Autodesk Inventor part; units mm, degrees
ref_plane "YZ Plane" through (0, 0, 0) normal (1, 0, 0) x (0, 1, 0)
ref_plane "XZ Plane" through (0, 0, 0) normal (0, 1, 0) x (-1, 0, 0)
ref_plane "XY Plane" through (0, 0, 0) normal (0, 0, 1) x (1, 0, 0)
sketch "Sketch1" plane through (0, 0, 0) normal (0, 0, 1) x (1, 0, 0)
  line L0 (-99.06, 38.1) -> (-99.06, -38.1)
  circle A0 centre (-60.96, 0) radius 12.7
  circle A1 centre (99.06, 0) radius 1.27
  line L1 (-99.06, 38.1) -> (99.06, 38.1)
  line L2 (-99.06, -38.1) -> (99.06, -38.1)
  arc A2 (99.06, -38.1) -> (99.06, 38.1) centre (99.06, 0) ccw
  line L3 (-48.6633, 3.175) -> (-45.3613, 3.175)
  line L4 (-45.3613, 3.175) -> (-45.3613, -3.175)
  line L5 (-45.3613, -3.175) -> (-48.6633, -3.175)
  point P0 (0, 0)
  point P1 (-99.06, 0)
  point P2 (106.7321, -3.216)
  point P3 (113.0654, -3.216)
  point P4 (-45.3613, 0)
  point P5 (0, -38.1)
  dimension "d0" = 76.2
  dimension "d4" = 25.4
  dimension "d13" = 2.54
  dimension "d14" = 6.35
  dimension "d15" = 160.02
  dimension "d16" = 3.302
  dimension "d17" = 38.1
extrude "Extrusion2" add sketch "Sketch1" along normal blind 25.4
sketch "Sketch2" plane through (0, 0, 25.4) normal (0, 0, 1) x (1, 0, 0)
  arc A0 (-48.6633, 3.175) -> (-48.6633, -3.175) centre (-60.96, 0) ccw
  point P0 (0, 0)
  point P1 (-80.01, 19.05)
  point P2 (-41.91, 19.05)
  point P3 (-41.91, -19.05)
  point P4 (-80.01, -19.05)
  dimension "d20" = 38.1
  dimension "d21" = 38.1
  dimension "d22" = 19.05
  dimension "d23" = 19.05
hole "Hole1" at (-80.01, 19.05, 25.4) at (-41.91, 19.05, 25.4) at (-41.91, -19.05, 25.4) at (-80.01, -19.05, 25.4) direction (0, 0, -1) diameter 4.9784 depth 25.4 tip angle 118
sketch "Sketch4" plane through (0, 0, 25.4) normal (0, 0, 1) x (1, 0, 0)
  circle A0 centre (99.06, 0) radius 1.27
  point P0 (0, 0)
hole "Hole3" at (99.06, 0, 25.4) direction (0, 0, -1) diameter 10.5918 end through all
properties part number "Motor_Arm"
Geometry check sheet. Reference: the model listing, model coordinates, mm. Coordinates: 2 decimals unless noted, no trailing zeros. Order: outer loops, then holes, each group sorted by start corner. A loop starts at its lowest first (then second) coordinate and runs counter-clockwise, first axis right, second up.
Item 1: Section check B-B (x = -60.96). Enter the section's corners in (y, z).
Item 2: Scan lines: line 1 along X through (y, z) = (0, 15.75); line 2 along Y through (x, z) = (99.06, 7.75); line 3 along X through (y, z) = (18.5, 7). Record each from-to range of solid material in increasing order.
Item 3: Section check D-D (y = 19.05). Enter the section's corners in (x, z).
Item 4: Section check C-C (z = 19.5). Enter the section's corners in (x, y) (3 decimals).
Item 5: Section check A-A (y = 0). Enter the section's corners in (x, z).
Item 6: Mould release check, pull along X, two halves, no side actions. Record for faces 1 (the flat face through (-99.06, 1, 13)), 2 (the flat face through (-45.361, 0, 13)), 3 (the flat face through (-1, -38.1, 13)): released by +X, released by -X, zero draft, split by the parting line, or undercut.
Check sheet entries:
1. outline: (-38.1, 0) - (-12.7, 0) - (-12.7, 25.4) - (-38.1, 25.4) - close; (12.7, 0) - (38.1, 0) - (38.1, 25.4) - (12.7, 25.4) - close
2. line 1: x = -99.06 to -73.66, -45.36 to 93.76, 104.36 to 137.16
2. line 2: y = -38.1 to -5.3, 5.3 to 38.1
2. line 3: x = -99.06 to -82.44, -77.58 to -44.34, -39.48 to 132.37
3. outline: (-99.06, 0) - (-82.5, 0) - (-82.5, 25.4) - (-99.06, 25.4) - close; (-77.52, 0) - (-44.4, 0) - (-44.4, 25.4) - (-77.52, 25.4) - close; (-39.42, 0) - (132.06, 0) - (132.06, 25.4) - (-39.42, 25.4) - close
4. outline: (-99.06, -38.1) - (99.06, -38.1) arc R38.1 ccw to (99.06, 38.1) - (-99.06, 38.1) - close; hole circle Ø4.978 at (-80.01, -19.05); hole circle Ø4.978 at (-80.01, 19.05); hole (-48.663, -3.175) - (-45.361, -3.175) - (-45.361, 3.175) - (-48.663, 3.175) arc R12.7 ccw (long way) to start; hole circle Ø4.978 at (-41.91, -19.05); hole circle Ø4.978 at (-41.91, 19.05); hole circle Ø10.592 at (99.06, 0)
5. outline: (-99.06, 0) - (-73.66, 0) - (-73.66, 25.4) - (-99.06, 25.4) - close; (-45.36, 0) - (93.76, 0) - (93.76, 25.4) - (-45.36, 25.4) - close; (104.36, 0) - (137.16, 0) - (137.16, 25.4) - (104.36, 25.4) - close
6. face 1: released by -X
6. face 2: undercut
6. face 3: zero draft
